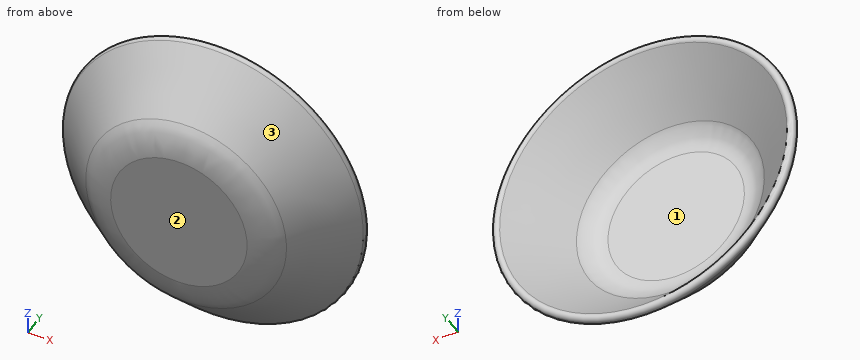
from build123d import *


with BuildPart() as part:
    # Sketch1 → Revolve1 (revolve)
    with BuildSketch(Plane.XY, mode=Mode.PRIVATE) as revolve1_sk:
        with BuildLine():
            Line((0, 0), (37.5, 0))
            ThreePointArc((37.5, 0), (47.067085809, 1.903011687), (55.17766953, 7.32233047))
            Line((55.17766953, 7.32233047), (82.5, 34.644660941))
            ThreePointArc((82.5, 34.644660941), (82.5, 38.180194847), (78.964466094, 38.180194847))
            Line((78.964466094, 38.180194847), (51.642135624, 10.857864376))
            ThreePointArc((51.642135624, 10.857864376), (45.153668647, 6.52240935), (37.5, 5))
            Line((37.5, 5), (0, 5))
            Line((0, 5), (0, 0))
        make_face()
    revolve(revolve1_sk.sketch.rotate(Axis((0, 0, 0), (0, 1, 0)), 90), axis=Axis((0, 0, 0), (0, 1, 0)))


solid = part.part
Could you check a few things on this model? Use its own coordinates, in mm. Face numbers are marked on the shaded views. Give positions to 0.01 mm unless a question says otherwise; leave off trailing zeros. Order: outer loops, then holes, each group sorted by start corner. A loop starts at its lowest first (then second) coordinate and runs counter-clockwise, first axis right, second up.
Item 1: If we section it at A-A, the plane x = 0: Write out the boundary of the cut face in (y, z), plus the area to 3 significant figures.
Item 2: I need wall thicknesses on line 1 (Z direction, x = 12, y = 28); line 2 (X direction, y = 35, z = 65.5); line 3 (X direction, y = 31.5, z = -36). Which ranges of each line are inside material? Lowest first, please.
Item 3: If we section it at C-C, the plane y = 29.5: Write out the boundary of the cut face in (x, z), plus the area to 3 significant figures.
Item 4: If we section it at B-B, the plane z = 0: Write out the boundary of the cut face in (x, y).
Item 5: I'm going to push flat-ended pins straight in: pin 1 (12 mm diameter, centred on x = -56.5, y = 30.5, fed in from -Z); pin 2 (6 mm diameter, centred on x = 41, z = 63, fed in from -Y); pin 3 (2 mm diameter, centred on x = -19, y = 8, fed in from -Z). Where does each tip first touch, or does it pass through?
Item 6: If we mould it in two halves opening along X, with no side actions, what happens to the marked faces 1, 2 and 3? For each: pulls with the +X half, pulls with the -X half, needs draft (parallel to the pull), parting line crosses it, or undercut.
Values:
1. outline: (0, -37.5) arc R25 ccw to (7.32, -55.18) - (34.64, -82.5) arc R2.5 ccw to (38.18, -78.96) - (10.86, -51.64) arc R20 cw to (5, -37.5) - (5, 37.5) arc R20 cw to (10.86, 51.64) - (38.18, 78.96) arc R2.5 ccw to (34.64, 82.5) - (7.32, 55.18) arc R25 ccw to (0, 37.5) - close
1. area: 958 mm2
2. line 1: z = -74.9 to -67.73, 67.73 to 74.9
2. line 2: x = -50.64 to -38.12, 38.12 to 50.64
2. line 3: x = -70.72 to -62.68, 62.68 to 70.72
3. outline: circle Ø154.71 at (0, 0); hole circle Ø140.57 at (0, 0)
3. area: 3,280 mm2
4. outline: (-82.5, 34.64) - (-55.18, 7.32) arc R25 ccw to (-37.5, 0) - (37.5, 0) arc R25 ccw to (55.18, 7.32) - (82.5, 34.64) arc R2.5 ccw to (78.96, 38.18) - (51.64, 10.86) arc R20 cw to (37.5, 5) - (-37.5, 5) arc R20 cw to (-51.64, 10.86) - (-78.96, 38.18) arc R2.5 ccw to start
5. pin 1: stops at z = -64
5. pin 2: stops at y = 24.31
5. pin 3: stops at z = -53.64
6. face 1: undercut
6. face 2: needs draft
6. face 3: parting line crosses it
